Verification items for the finished model (mm, model axes). A direction names the side the tool comes from. Round coordinates to 2 decimals unless told otherwise and drop trailing zeros. Order: outer loops, then holes, each group sorted by start corner. A loop starts at its lowest first (then second) coordinate and runs counter-clockwise, first axis right, second up. Notation, with made-up numbers: (20.5, 65.5) -> (37.5, 65.5) arc R18 ccw to (37.5, 94.5) -> close; hole circle Ø1 at (33.25, 48). An arc over 180 degrees is marked (long way). Put each result on its own line as item: value.
```python
from build123d import *

# Parameters (mm, degrees)
SKETCH_1_W               = 85
SKETCH_1_H               = 60
SKETCH_1_R               = 25
EXTRUDE_1_DEPTH          = 6
PATTERN_CIRCULAR_1_COUNT = 4
CUT_EXTRUDE_1_DEPTH      = 6
CHAMFER_1_SIZE           = 2


with BuildPart() as part:
    # 草图1 → 凸台-拉伸1 (new body)
    with BuildSketch(Plane.XY):
        Rectangle(SKETCH_1_W, SKETCH_1_H)
        Circle(SKETCH_1_R, mode=Mode.SUBTRACT)
    extrude(amount=EXTRUDE_1_DEPTH)

    # 草图2 → M4 螺纹孔1 (revolve, cut)
    with BuildSketch(Plane(origin=(24.748737342, 24.748737342, 6), x_dir=(0, -1, 0), z_dir=(1, 0, 0))):
        Polygon((0, 0), (0, 12.491420021), (1.65, 11.5), (1.65, 0), align=None)
    hole_wizard_m4_1 = revolve(axis=Axis((24.748737342, 24.748737342, 12.35), (0, 0, -1)), mode=Mode.SUBTRACT)

    # 阵列(圆周)1: M4 螺纹孔1 ×4 about axis
    pattern_circular_1_axis = Axis((0, 0, 0), (0, 0, 1))
    for i in range(1, PATTERN_CIRCULAR_1_COUNT):
        add(hole_wizard_m4_1.rotate(pattern_circular_1_axis, i * 360 / PATTERN_CIRCULAR_1_COUNT), mode=Mode.SUBTRACT)

    # 草图4 → 切除-拉伸1 (cut)
    with BuildSketch(Plane.XY.offset(6)):
        with BuildLine():
            Line((40.2, 24), (40.2, 16))
            ThreePointArc((40.2, 16), (37.5, 13.3), (34.8, 16))
            Line((34.8, 16), (34.8, 24))
            ThreePointArc((34.8, 24), (37.5, 26.7), (40.2, 24))
        make_face()
        with BuildLine():
            Line((40.2, -24), (40.2, -16))
            ThreePointArc((40.2, -16), (37.5, -13.3), (34.8, -16))
            Line((34.8, -16), (34.8, -24))
            ThreePointArc((34.8, -24), (37.5, -26.7), (40.2, -24))
        make_face()
        with BuildLine():
            Line((-40.2, 24), (-40.2, 16))
            ThreePointArc((-40.2, 16), (-37.5, 13.3), (-34.8, 16))
            Line((-34.8, 16), (-34.8, 24))
            ThreePointArc((-34.8, 24), (-37.5, 26.7), (-40.2, 24))
        make_face()
        with BuildLine():
            Line((-40.2, -24), (-40.2, -16))
            ThreePointArc((-40.2, -16), (-37.5, -13.3), (-34.8, -16))
            Line((-34.8, -16), (-34.8, -24))
            ThreePointArc((-34.8, -24), (-37.5, -26.7), (-40.2, -24))
        make_face()
    extrude(amount=-CUT_EXTRUDE_1_DEPTH, mode=Mode.SUBTRACT)

    # 倒角1
    chamfer_1_edges = [part.edges().sort_by_distance(p)[0] for p in [
        (42.5, -30, 3),
        (-42.5, -30, 3),
        (-42.5, 30, 3),
        (42.5, 30, 3),
    ]]
    chamfer(chamfer_1_edges, length=CHAMFER_1_SIZE)


solid = part.part
```
Item 1: Release check for a two-part mould opening along X. For faces 3 (the face through (42.5, 0, 3)), 4 (the face through (-1, 27, 6)), 5 (the face through (37.4, 26.7, 3)), 6 (the face through (-23.987, 26.213, 3.042)) record: pulls with the +X half, pulls with the -X half, needs draft (parallel to the pull), parting line crosses it, or undercut.
Geometry check:
face 3: pulls with the +X half
face 4: needs draft
face 5: undercut
face 6: undercut
Item 2: Material ranges on line 1 along X through (y, z) = (22, 3.2); line 2 along X through (y, z) = (25.5, 4.45) (3 decimals); line 3 along Y through (x, z) = (35.5, 5.05), recorded low to high.
Geometry check:
line 1: -42.5 to -40.2, -34.8 to -11.87, 11.87 to 34.8, 40.2 to 42.5
line 2: -42.5 to -39.745, -35.255 to -26.218, -23.28 to 23.28, 26.218 to 35.255, 39.745 to 42.5
line 3: -30 to -25.81, -14.19 to 14.19, 25.81 to 30
Item 3: Sectioned sample at D-D, the plane y = 19. Record the boundary of the cut face in (x, z), then the cut area to 3 significant figures.
Geometry check:
outline: (-42.5, 0) -> (-40.2, 0) -> (-40.2, 6) -> (-42.5, 6) -> close; (-34.8, 0) -> (-16.25, 0) -> (-16.25, 6) -> (-34.8, 6) -> close; (16.25, 0) -> (34.8, 0) -> (34.8, 6) -> (16.25, 6) -> close; (40.2, 0) -> (42.5, 0) -> (42.5, 6) -> (40.2, 6) -> close
area: 250 mm2
Item 4: Sectioned sample at A-A, the plane x = -37.5. Record the boundary of the cut face in (y, z), then the cut area to 3 significant figures.
Geometry check:
outline: (-30, 0) -> (-26.7, 0) -> (-26.7, 6) -> (-30, 6) -> close; (-13.3, 0) -> (13.3, 0) -> (13.3, 6) -> (-13.3, 6) -> close; (26.7, 0) -> (30, 0) -> (30, 6) -> (26.7, 6) -> close
area: 199 mm2
Item 5: Sectioned sample at B-B, the plane y = -7. Record the boundary of the cut face in (x, z), then the cut area to 3 significant figures.
Geometry check:
outline: (-42.5, 0) -> (-24, 0) -> (-24, 6) -> (-42.5, 6) -> close; (24, 0) -> (42.5, 0) -> (42.5, 6) -> (24, 6) -> close
area: 222 mm2
Item 6: Tool access check on faces 1 (the face through (-42.5, 0, 3)), 2 (the face through (-34.8, 20, 3)). Record the directions out of +Z, -Z, +X, -X, +Y, -Y that give a thin tool (end or side, any length) a straight path to the whole face; none if there is none.
Geometry check:
face 1: +Z, -Z, -X, +Y, -Y
face 2: +Z, -Z
Item 7: Depth check by flat-ended pin: pin 1 Ø3 at (x, y) = (24.75, -24.75) entering from -Z. Enter the tip coordinate at first touch or a pass-through.
Geometry check:
pin 1: through
Item 8: Sectioned sample at C-C, the plane x = -3.5. Record the boundary of the cut face in (y, z), then the cut area to 3 significant figures.
Geometry check:
outline: (-30, 0) -> (-24.75, 0) -> (-24.75, 6) -> (-30, 6) -> close; (24.75, 0) -> (30, 0) -> (30, 6) -> (24.75, 6) -> close
area: 63.0 mm2
